The figure shows three views and two pictorial views of one solid part (mm, origin at its lowest corner). Answer the questions. A direction names the side the tool comes from. Coordinates: 2 decimals unless noted, no trailing zeros. Loops run counter-clockwise (first coordinate to the right, second up) from the corner with the lowest first, then second, coordinate; pieces in that order, holes last. Notation, with made-up numbers: M 83,-18.75 L 98,-18.75 A26 ccw 98,10.25 Z; hole C 35,8 d3. An arc over 180 degrees is marked long. One line per item, written item: value. Start each with the question number.
1. The part is cut by section A-A (y = 18.25). Write down the section's boundary in (x, z).
2. The part is cut by section C-C (x = 32). Write down the section's boundary in (y, z).
3. For the marked faces 1 and 2, determine the directions among +Z, -Z, +X, -X, +Y, -Y from which every point of the face is accessible in a straight line to the end or side of a thin tool.
4. Flat-ended cylindrical pins translate along their axes: pin 1 (12 mm diameter, centred on y = 30, z = 13, fed in from +X); pin 2 (4 mm diameter, centred on x = 7, z = 6.5, fed in from -Y); pin 3 (12 mm diameter, centred on x = 11.5, y = 24.5, fed in from -Z). Find the tip coordinate at first contact, or state that the pin passes through.
5. Consider probe 1 along Z at (x, y) = (40, 18.5); probe 2 along X at (y, z) = (19.5, 9.5). Determine where each line is inside the solid, lowest interval first.
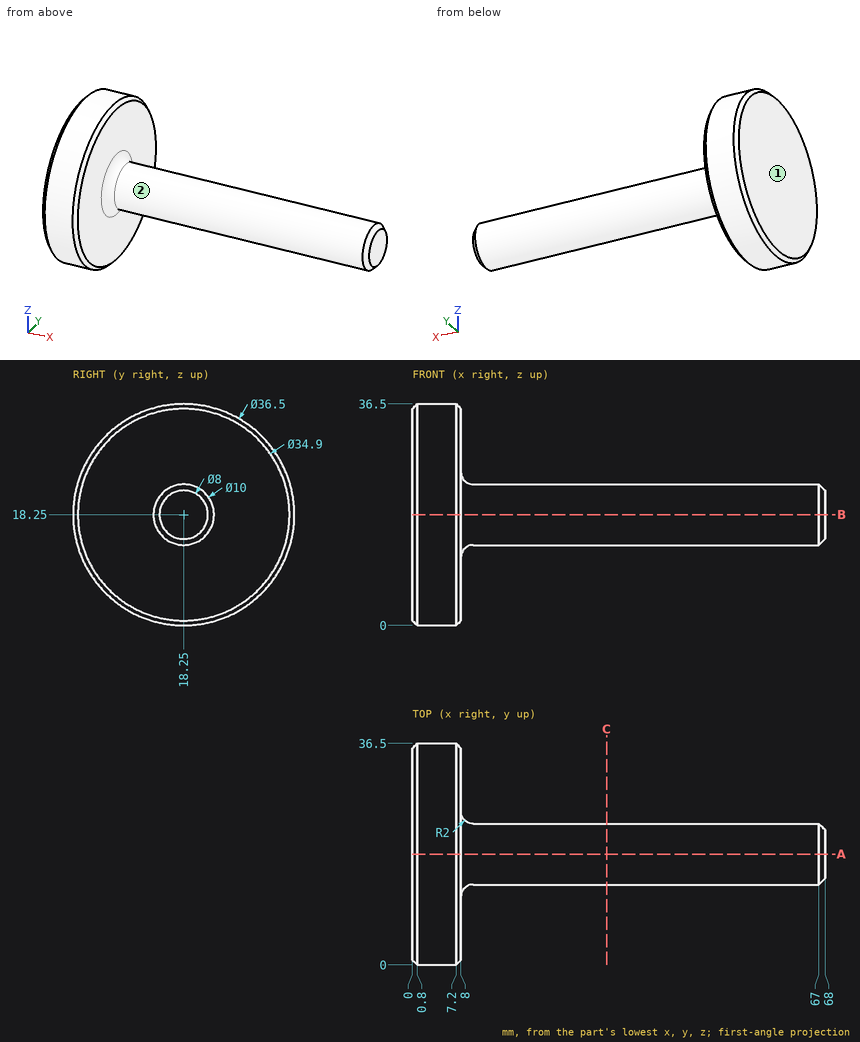
Answer block:
1. outline: M 0,0.8 L 0.8,0 L 7.2,0 L 8,0.8 L 8,11.25 A2 cw 10,13.25 L 67,13.25 L 68,14.25 L 68,22.25 L 67,23.25 L 10,23.25 A2 cw 8,25.25 L 8,35.7 L 7.2,36.5 L 0.8,36.5 L 0,35.7 Z
2. outline: C 18.25,18.25 d10
3. face 1: +Z, -Z, -X, +Y, -Y
3. face 2: +X
4. pin 1: stops at x = 8
4. pin 2: stops at y = 2.82
4. pin 3: stops at z = 0.12
5. probe 1: z = 13.26 to 23.24
5. probe 2: x = 0 to 8
